Geometry: final body of the model. Coordinates: model frame, mm. Face numbers are marked on the shaded views. A direction names the side the tool comes from. Round coordinates to 2 decimals unless told otherwise and drop trailing zeros. Loops run counter-clockwise (first coordinate to the right, second up) from the corner with the lowest first, then second, coordinate; pieces in that order, holes last. Notation, with made-up numbers: (12.5, 32) - (44.5, 32) arc R17 cw to (44.5, 62) - close; hole circle Ø10 at (-21.5, 55.5). An arc over 180 degrees is marked (long way). Answer as a JSON object with one key per item and string values. Group by question number.
Item 1: Draft query along Z for the marked faces 3, 4 and 5. Return one class per face: released by +Z, released by -Z, zero draft, split by the parting line, or undercut.
Item 2: Section A-A (x = -16). Return the cut outline in (y, z).
Item 3: Line query: line 1 (X direction, y = 25, z = 5); line 2 (Y direction, x = 15.65, z = -41.5); line 3 (X direction, y = 19.75, z = -16). Output: solid intervals per line, ascending.
Item 4: Reachability of the marked faces 1 and 2 from +Z, -Z, +X, -X, +Y, -Y: full face, straight path, thin tool, end or side. Return the list, or none.
Item 5: First-contact query: pin 1 (3 mm diameter, centred on x = 16, z = -10, fed in from -Y); pin 2 (6 mm diameter, centred on x = -9.5, z = -35, fed in from +Y); pin 3 (4.5 mm diameter, centred on y = 11.5, z = 9.5, fed in from -X); pin 4 (3 mm diameter, centred on y = 15.5, z = -24, fed in from +X). Flat tips, straight axial feed; report the tip coordinate or a pass-through.
Item 6: Section B-B (z = -10). Return the cut outline in (x, y), plus the area to 3 significant figures.
Item 7: Section C-C (y = 5). Return the cut outline in (x, z).
Item 8: Section D-D (z = 5). Return the cut outline in (x, y).
```python
from build123d import *

# Parameters (mm, degrees)
SKETCH_W             = 64
SKETCH_H             = 54
PAD_DEPTH            = 27
POCKET_DEPTH         = 24
SKETCH002_R          = 2.1
POCKET001_DEPTH      = 3
SKETCH003_R          = 7
POCKET002_DEPTH      = 3
SKETCH004_R          = 2
PAD001_DEPTH         = 5
SKETCH011_R          = 2
POCKET006_DEPTH      = 3
BODY_PITCH_ANGLE     = -90
BODY_PLACEMENT_ANGLE = -90


with BuildPart() as part:
    # Sketch → Pad (new body)
    with BuildSketch(Plane.XY):
        with Locations((20, 15)):
            Rectangle(SKETCH_W, SKETCH_H)
    extrude(amount=-PAD_DEPTH)

    # Sketch001 (on Face5 of Pad) → Pocket (cut)
    with BuildSketch(Plane.XY):
        Polygon((-9, 32), (-9, 39), (49, 39), (49, 32), (40.5, 32), (40.5, 29), (49, 29), (49, -9), (-9, -9), (-9, 29), (-0.5, 29), (-0.5, 32), align=None)
    extrude(amount=-POCKET_DEPTH, mode=Mode.SUBTRACT)

    # Sketch002 (on Face16 of Pocket) → Pocket001 (cut)
    with BuildSketch(Plane.XZ.offset(-29)):
        with Locations((45.3, -5.5)):
            Circle(SKETCH002_R)
        with Locations((45.3, -14.5)):
            Circle(SKETCH002_R)
        with Locations((-5, -5.5)):
            Circle(SKETCH002_R)
        with Locations((-5, -14.5)):
            Circle(SKETCH002_R)
    extrude(amount=-POCKET001_DEPTH, mode=Mode.SUBTRACT)

    # Sketch003 (on Face1 of Pocket001) → Pocket002 (cut)
    with BuildSketch(Plane(origin=(0, 42, 0), x_dir=(-1, 0, 0), z_dir=(0, 1, 0))):
        with Locations((-10, -10)):
            Circle(SKETCH003_R)
    extrude(amount=-POCKET002_DEPTH, mode=Mode.SUBTRACT)

    # Sketch004 (on Face7 of Pocket002) → Pad001 (join)
    with BuildSketch(Plane.XZ.offset(12)):
        with Locations((10, -10)):
            Circle(SKETCH004_R)
    extrude(amount=PAD001_DEPTH)

    # Sketch011 (on Face5 of Pocket) → Pocket006 (cut)
    with BuildSketch(Plane(origin=(0, 0, -27), x_dir=(1, 0, 0), z_dir=(0, 0, -1))):
        with Locations((26.5, 1)):
            Circle(SKETCH011_R)
        with Locations((10.5, 1)):
            Circle(SKETCH011_R)
        with Locations((26.5, -31)):
            Circle(SKETCH011_R)
        with Locations((10.5, -31)):
            Circle(SKETCH011_R)
    extrude(amount=-POCKET006_DEPTH, mode=Mode.SUBTRACT)


with BuildPart() as part_1:
    # Body pitch: moved
    add(part.part.rotate(Axis((0, 0, 0), (0, 1, 0)), BODY_PITCH_ANGLE))


with BuildPart() as part_2:
    # Body placement: moved
    add(part_1.part.moved(Location((-15, 27, -36.5))).rotate(Axis((-15, 27, -36.5), (0, 0, 1)), BODY_PLACEMENT_ANGLE))


solid = part_2.part
```
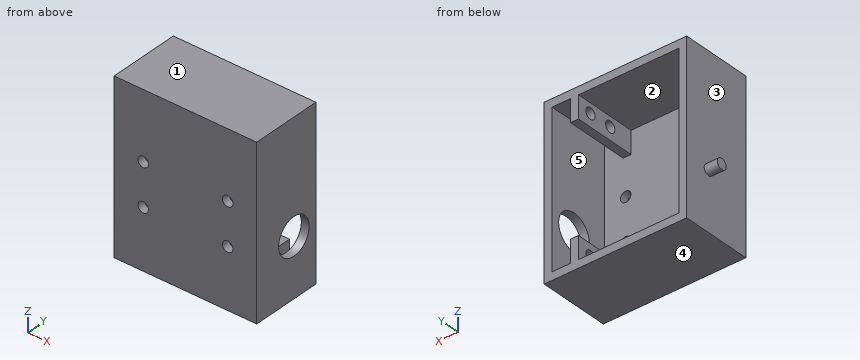
Values:
{
 "1": {"face 3": "zero draft", "face 4": "released by -Z", "face 5": "undercut"},
 "2": {"outline": "(0, -48.5) - (27, -48.5) - (27, -45.5) - (3, -45.5) - (3, -28) - (0, -28) - close; (0, -24) - (3, -24) - (3, -12) - (0, -12) - close; (0, -8) - (3, -8) - (3, 12.5) - (27, 12.5) - (27, 15.5) - (0, 15.5) - close"},
 "3": {"line 1": "x = -27 to -24, 14 to 17, 24 to 27", "line 2": "y = 0 to 10.4, 14.6 to 19.4, 23.6 to 27", "line 3": "x = -27 to -24, 24 to 27"},
 "4": {"face 1": "+Z, +X, -X, +Y, -Y", "face 2": "+Y"},
 "5": {"pin 1": "passes through", "pin 2": "stops at y = 3", "pin 3": "stops at x = -27", "pin 4": "stops at x = -24"},
 "6": {"outline": "(-27, 0) - (-18, 0) - (-18, 3) - (-24, 3) - (-24, 27) - (-27, 27) - close; (-14, 0) - (14, 0) - (14, 3) - (-14, 3) - close; (18, 0) - (27, 0) - (27, 27) - (24, 27) - (24, 3) - (18, 3) - close", "area": "282 mm^2"},
 "7": {"outline": "(-27, -48.5) - (27, -48.5) - (27, 15.5) - (-27, 15.5) - close; hole (-24, -45.5) - (14, -45.5) - (14, -37) - (17, -37) - (17, -45.5) - (24, -45.5) - (24, 12.5) - (17, 12.5) - (17, 4) - (14, 4) - (14, 12.5) - (-24, 12.5) - close"},
 "8": {"outline": "(-27, 0) - (27, 0) - (27, 27) - (24, 27) - (24, 3) - (17, 3) - (17, 27) - (14, 27) - (14, 3) - (-24, 3) - (-24, 27) - (-27, 27) - close"}
}
